Verification items for the finished model (mm, model axes). A direction names the side the tool comes from. Coordinates: 2 decimals unless noted, no trailing zeros. Write each loop counter-clockwise with the first axis right and the second up, starting at its lowest first coordinate (ties: lowest second). Pieces come first, ordered by that corner, then holes. Notation, with made-up numbers: M -31.5,59.25 L -1.5,59.25 A22 cw -1.5,65.25 Z; hole C 4.5,6 d11. An arc over 180 degrees is marked long. One line per item, written item: value.
```python
from build123d import *

# Parameters (mm, degrees)
BOSS_EXTRU_1_DEPTH      = 10
ENL_V_MAT_EXTRU_3_DEPTH = 129.452325787


with BuildPart() as part:
    # Esquisse1 → Boss.-Extru.1 (new body)
    with BuildSketch(Plane.XY):
        with BuildLine():
            Line((0, 0), (80, 0))
            ThreePointArc((80, 0), (100, 20), (80, 40))
            ThreePointArc((80, 40), (100, 60), (80, 80))
            Line((80, 80), (0, 80))
            Line((0, 80), (0, 0))
        make_face()
        with BuildLine():
            Line((72, 8), (72, 32))
            Line((72, 32), (80, 32))
            ThreePointArc((80, 32), (92, 20), (80, 8))
            Line((80, 8), (72, 8))
        make_face(mode=Mode.SUBTRACT)
        with BuildLine():
            Line((72, 48), (80, 48))
            ThreePointArc((80, 48), (92, 60), (80, 72))
            Line((80, 72), (72, 72))
            Line((72, 72), (72, 48))
        make_face(mode=Mode.SUBTRACT)
    extrude(amount=BOSS_EXTRU_1_DEPTH)

    # Esquisse2 → Enlèv. mat.-Extru.3 (cut, through all)
    with BuildSketch(Plane.XY.offset(10)):
        Polygon((49.85041269, 44.450222472), (41.772697951, 58.441234808), (25.617268474, 58.441234808), (17.539553736, 44.450222472), (25.617268474, 30.459210135), (41.772697951, 30.459210135), align=None)
    extrude(amount=-ENL_V_MAT_EXTRU_3_DEPTH, mode=Mode.SUBTRACT)


solid = part.part
```
Item 1: Cross-section at B-B, the plane z = 3.25. Enter the section's corners in (x, y), and give its area (3 significant figures).
The answers:
outline: M 0,0 L 80,0 A20 ccw 80,40 A20 ccw 80,80 L 0,80 Z; hole M 17.54,44.45 L 25.62,30.46 L 41.77,30.46 L 49.85,44.45 L 41.77,58.44 L 25.62,58.44 Z; hole M 72,8 L 80,8 A12 ccw 80,32 L 72,32 Z; hole M 72,48 L 80,48 A12 ccw 80,72 L 72,72 Z
area: 6,140 mm²
Item 2: Cross-section at D-D, the plane y = 33.5. Enter the section's corners in (x, z).
The answers:
outline: M 0,0 L 23.86,0 L 23.86,10 L 0,10 Z; M 43.53,0 L 94.76,0 L 94.76,10 L 43.53,10 Z
Item 3: Go/stop test with flat-tipped pins: P1, Ø5, axis at y = 44.5, z = 4.5, coming from the +X side; P2, Ø2, axis at y = 49.5, z = 4.5, coming from the +X side. Record where each tip stops, or that it passes through.
The answers:
P1: stops at x = 95.2
P2: stops at x = 97.6
Item 4: Access from +Z, -Z, +X, -X, +Y, -Y to the whole of each face (thin tool, end or side, straight path). Record for faces 4 (the face through (0, 41, 5)), 5 (the face through (45.755, 37.357, 5.07)).
The answers:
face 4: +Z, -Z, -X, +Y, -Y
face 5: +Z, -Z
Item 5: Scan lines: line 1 (Y direction, x = 74.5, z = 0.75); line 2 (X direction, y = 53, z = 5) (3 decimals); line 3 (Y direction, x = 96, z = 8.75). Record each from-to range of solid material in increasing order.
The answers:
line 1: y = 0 to 8, 32 to 48, 72 to 80
line 2: x = 0 to 22.476, 44.914 to 72, 89.747 to 98.735
line 3: y = 8 to 32, 48 to 72
Item 6: Cross-section at A-A, the plane y = 20. Enter the section's corners in (x, z).
The answers:
outline: M 0,0 L 72,0 L 72,10 L 0,10 Z; M 92,0 L 100,0 L 100,10 L 92,10 Z
Item 7: Draft check along Y on faces 1 (the face through (76, 32, 5)), 2 (the face through (41, 80, 5)), 3 (the face through (49, 41, 10)). Enter one of: released by +Y, released by -Y, zero draft, split by the parting line, or undercut.
The answers:
face 1: undercut
face 2: released by +Y
face 3: zero draft
Item 8: Cross-section at C-C, the plane x = 83.5. Enter the section's corners in (y, z), and give its area (3 significant figures).
The answers:
outline: M 0.31,0 L 8.52,0 L 8.52,10 L 0.31,10 Z; M 31.48,0 L 39.69,0 L 39.69,10 L 31.48,10 Z; M 40.31,0 L 48.52,0 L 48.52,10 L 40.31,10 Z; M 71.48,0 L 79.69,0 L 79.69,10 L 71.48,10 Z
area: 329 mm²
